Drawing for the job (mm, zero at the part's lowest x, y, z). A direction names the side the tool comes from. Give positions to 0.01 mm unless a question says otherwise; leave off trailing zeros. Write each loop counter-clockwise with the first axis right and the second up, starting at its lowest first coordinate (ties: lowest second). Pieces come first, ordered by that corner, then holes. Notation, with made-up numbers: M 74.25,-20.75 L 85.25,-20.75 A20 cw 85.25,16.25 Z; hole C 62,46 d5. An arc over 180 degrees is marked long. Use a Markdown table: item, result. Add a question column.
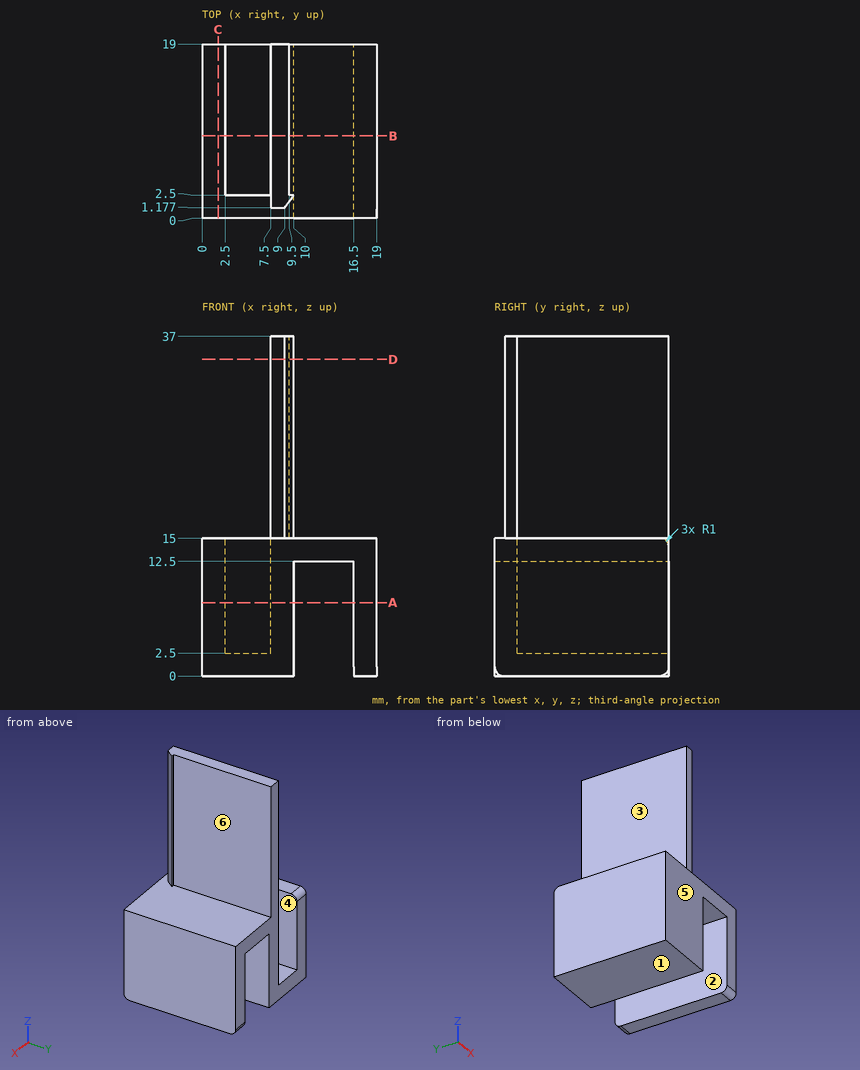
1. Flat gauge pins, fed straight in: pin 1 (2.5 mm diameter, centred on x = 6, z = 6.5, fed in from +Y); pin 2 (2 mm diameter, centred on x = 14, y = 8.5, fed in from -Z); pin 3 (5.5 mm diameter, centred on x = 4, y = 9.5, fed in from +Z). Where does each tip first touch, or does it go through?
2. Cut at C-C (x = 1.75). Write the cut outline in (y, z).
3. Mould opens along X. For the marked faces 4, 5 and 6 say: released by +X, released by -X, zero draft, split by the parting line, or undercut.
4. Cut at A-A (z = 8). Write the cut outline in (x, y).
5. Tool access for the marked faces 1, 2 and 3: list every direction of +Z, -Z, +X, -X, +Y, -Y with a clear straight run to the whole face (end or side of a thin tool).
6. Cut at B-B (y = 9). Write the cut outline in (x, z).
7. Drill centre lines: probe 1 along X at (y, z) = (8.25, 4.5); probe 2 along X at (y, z) = (3.75, 13.5); probe 3 along X at (y, z) = (12.5, 32). Where is each one in solid material? Low to high. Write a range as [from, to].
8. Cut at D-D (z = 34.5). Write the cut outline in (x, y).
A:
| question | item | result |
|---|---|---|
| 1 | pin 1 | stops at y = 2.5 |
| 1 | pin 2 | stops at z = 12.5 |
| 1 | pin 3 | stops at z = 15 |
| 2 | outline | M 0,0 L 19,0 L 19,14 A1 ccw 18,15 L 0,15 Z |
| 3 | face 4 | undercut |
| 3 | face 5 | zero draft |
| 3 | face 6 | released by +X |
| 4 | outline | M 0,0 L 10,0 L 10,19 L 7.5,19 L 7.5,2.5 L 2.5,2.5 L 2.5,19 L 0,19 Z; M 16.5,0 L 19,0 L 19,19 L 16.5,19 Z |
| 5 | face 1 | -Z, +X, -X, +Y, -Y |
| 5 | face 2 | -Z, +Y, -Y |
| 5 | face 3 | +Z, +Y |
| 6 | outline | M 0,0 L 10,0 L 10,12.5 L 16.5,12.5 L 16.5,0 L 19,0 L 19,15 L 9.5,15 L 9.5,37 L 7.5,37 L 7.5,2.5 L 2.5,2.5 L 2.5,15 L 0,15 Z |
| 7 | probe 1 | x = [0, 2.5], [7.5, 10], [16.5, 19] |
| 7 | probe 2 | x = [0, 2.5], [7.5, 19] |
| 7 | probe 3 | x = [7.5, 9.5] |
| 8 | outline | M 7.5,1.18 L 9,1.18 L 10,2.5 L 9.5,2.5 L 9.5,19 L 7.5,19 Z |
